Autodesk Inventor part; units mm, degrees
ref_plane "YZ Plane" through (0, 0, 0) normal (1, 0, 0) x (0, 1, 0)
ref_plane "XZ Plane" through (0, 0, 0) normal (0, 1, 0) x (-1, 0, 0)
ref_plane "XY Plane" through (0, 0, 0) normal (0, 0, 1) x (1, 0, 0)
sketch "Sketch1" plane through (0, 0, 0) normal (1, 0, 0) x (0, 1, 0)
  line L0 (0, 0) -> (14, 0)
  line L1 (14, 0) -> (14, -30)
  line L2 (14, -30) -> (0, -30)
  line L3 (0, -30) -> (0, 0)
  line L4 (14, -30) -> (0, -30)
  line L5 (0, -30) -> (0, -30)
  line L6 (0, -30) -> (14, -30)
  line L7 (14, -30) -> (14, -30)
  line L8 (0, 0) -> (0, -18)
  line L9 (0, -18) -> (14, -18)
  line L10 (14, -18) -> (14, 0)
  point P0 (14, -18)
  dimension "d12" = 14
  dimension "d13" = 30
  dimension "d14" = 12
  dimension "d15" = 0
extrude "Extrusion6" add sketch "Sketch1" along normal blind 10 contours L9 L1 L2 L3
extrude "Extrusion7" add sketch "Sketch1" along normal blind 10 and the other way blind 18 contours L0 L1 L9 L3
fillet "Fillet2" radius 5 1 edges at (-18, 7, -18)
sketch "Sketch7" plane through (10, 0, 0) normal (1, 0, 0) x (0, 0, -1)
  line L0 (35, 14) -> (-6, 14)
  line L1 (-6, 14) -> (-6, 0)
  line L2 (-6, 0) -> (35, 0)
  line L3 (35, 0) -> (35, 14)
  line L4 (30, 0) -> (30, 14)
  circle A0 centre (32, 7) radius 1.5
  circle A1 centre (-3, 7) radius 1.5
  point P0 (0, 0)
  dimension "d32" = 41
  dimension "d33" = 5
  dimension "d34" = 14
  dimension "d35" = 3
  dimension "d36" = 3
  dimension "d37" = 3
  dimension "d38" = 35
extrude "Extrusion9" add sketch "Sketch7" along normal blind 6
properties part number "_3DPrint"
CAD build for the part. Positions are in the model's coordinates, mm. A direction names the side the tool comes from. Give positions to 0.01 mm unless a question says otherwise; leave off trailing zeros. Order: outer loops, then holes, each group sorted by start corner. A loop starts at its lowest first (then second) coordinate and runs counter-clockwise, first axis right, second up.
(1) Saw through at C-C, the plane x = 13.5. Give the cut face in (y, z), then the cut area to 3 significant figures.
(2) Drill centre lines: L1, parallel to Y at x = 13, z = 3; L2, parallel to Z at x = 1, y = 12.5; L3, parallel to X at y = 5, z = 2. Where is each one in solid material? Low to high.
(3) Mould opens along Z. For faces 4 (the flat face through (-7, 7, -18)), 5 (the flat face through (16, 7, -14)), 6 (the flat face through (-4, 7, 0)), 7 (the cylindrical face through (12.96, 8.33, 2.31)) say: released by +Z, released by -Z, zero draft, split by the parting line, or undercut.
(4) Tool access for faces 1 (the flat face through (3, 0, -10)), 2 (the flat face through (10, 9, 3)), 3 (the flat face through (5, 7, -30)): list every direction of +Z, -Z, +X, -X, +Y, -Y with a clear straight run to the whole face (end or side of a thin tool).
(5) Saw through at A-A, the plane z = 3. Give the cut face in (x, y), then the cut area to 3 significant figures.
(6) Saw through at D-D, the plane y = 9.5. Give the cut face in (x, z).
(7) Saw through at B-B, the plane y = 7. Give the cut face in (x, z).
(8) Flat gauge pins, fed straight in: pin 1 (5.5 mm diameter, centred on y = 6, z = -32, fed in from -X); pin 2 (7 mm diameter, centred on x = -4.5, y = 8.5, fed in from +Z); pin 3 (5 mm diameter, centred on y = 7, z = 3, fed in from -X); pin 4 (2 mm diameter, centred on x = -11, z = -11, fed in from -Y). Where does each tip first touch, or does it go through?
Results found:
1. outline: (0, -35) - (14, -35) - (14, 6) - (0, 6) - close; hole circle Ø3 at (7, -32); hole circle Ø3 at (7, 3)
1. area: 560 mm2
2. L1: y = 0 to 5.5, 8.5 to 14
2. L2: z = -30 to 0
2. L3: x = 10 to 16
3. face 4: released by -Z
3. face 5: zero draft
3. face 6: released by +Z
3. face 7: undercut
4. face 1: +Z, -Z, +X, -X, -Y
4. face 2: +Z, -X, +Y, -Y
4. face 3: -Z, -X, +Y, -Y
5. outline: (10, 0) - (16, 0) - (16, 5.5) - (10, 5.5) - close; (10, 8.5) - (16, 8.5) - (16, 14) - (10, 14) - close
5. area: 66.0 mm2
6. outline: (-18, -13) arc R5 ccw to (-13, -18) - (0, -18) - (0, -30) - (10, -30) - (10, -35) - (16, -35) - (16, 6) - (10, 6) - (10, 0) - (-18, 0) - close
7. outline: (-18, -13) arc R5 ccw to (-13, -18) - (0, -18) - (0, -30) - (10, -30) - (10, -30.5) - (16, -30.5) - (16, 1.5) - (10, 1.5) - (10, 0) - (-18, 0) - close; (10, -35) - (16, -35) - (16, -33.5) - (10, -33.5) - close; (10, 4.5) - (16, 4.5) - (16, 6) - (10, 6) - close
8. pin 1: stops at x = 0
8. pin 2: stops at z = 0
8. pin 3: stops at x = 10
8. pin 4: stops at y = 0
